Input: part model. Units: mm. Frame: model coordinates. Face numbers are marked on the shaded views. Round coordinates to 2 decimals unless told otherwise and drop trailing zeros. Write each loop counter-clockwise with the first axis right and the second up, starting at its lowest first coordinate (ties: lowest second). Pieces come first, ordered by that corner, then holes. Notation, with made-up numbers: (21.5, 81) -> (30.5, 81) arc R25 cw to (30.5, 97) -> close; hole circle Ø11 at (69, 5.5). An arc over 180 degrees is marked (long way). Use CSV: the item, a comma, the result in double quotes.
```python
from build123d import *

# Parameters (mm, degrees)
BOSS_EXTRUDE1_DEPTH     = 2.8
SKETCH3_W               = 25
SKETCH3_H               = 40
CUT_EXTRUDE1_DEPTH      = 1
SKETCH4_W               = 2.8
SKETCH4_H               = 15
BOSS_EXTRUDE2_DEPTH     = 15
CUT_EXTRUDE2_DEPTH      = 76.211967133
CUT_EXTRUDE2_DEPTH_BACK = 76.211967133
SKETCH5_R               = 2.5


with BuildPart() as part:
    # Sketch2 → Boss-Extrude1 (new body)
    with BuildSketch(Plane(origin=(0, 0, 0), x_dir=(1, 0, 0), z_dir=(0, 1, 0))):
        Polygon((-15, 27.5), (15, 27.5), (15, 7.5), (5, 7.5), (5, 0), (25, 0), (25, -60), (-25, -60), (-25, 0), (-5, 0), (-5, 7.5), (-15, 7.5), align=None)
    extrude(amount=BOSS_EXTRUDE1_DEPTH)

    # Sketch3 → Cut-Extrude1 (cut)
    with BuildSketch(Plane(origin=(0, 2.8, 0), x_dir=(1, 0, 0), z_dir=(0, 1, 0))):
        with Locations((0, -32.5)):
            Rectangle(SKETCH3_W, SKETCH3_H)
    extrude(amount=-CUT_EXTRUDE1_DEPTH, mode=Mode.SUBTRACT)

    # Sketch4 → Boss-Extrude2 (add)
    with BuildSketch(Plane.XZ):
        with Locations((16.4, 30)):
            Rectangle(SKETCH4_W, SKETCH4_H)
        with Locations((-16.4, 30)):
            Rectangle(SKETCH4_W, SKETCH4_H)
    extrude(amount=BOSS_EXTRUDE2_DEPTH)

    # Sketch5 → Cut-Extrude2 (cut, two sides: drawn at the far end of the back side and taken through both)
    with BuildSketch(Plane(origin=(17.8, 0, 0), x_dir=(0, 0, -1), z_dir=(1, 0, 0)).offset(-CUT_EXTRUDE2_DEPTH_BACK)):
        with Locations((-30, -7.5)):
            Circle(SKETCH5_R)
        with BuildLine():
            Line((-22.5, -16.5), (-37.5, -16.5))
            Line((-37.5, -16.5), (-37.5, -7.5))
            ThreePointArc((-37.5, -7.5), (-30, -15), (-22.5, -7.5))
            Line((-22.5, -7.5), (-22.5, -16.5))
        make_face()
    extrude(amount=CUT_EXTRUDE2_DEPTH + CUT_EXTRUDE2_DEPTH_BACK, mode=Mode.SUBTRACT)


solid = part.part
```
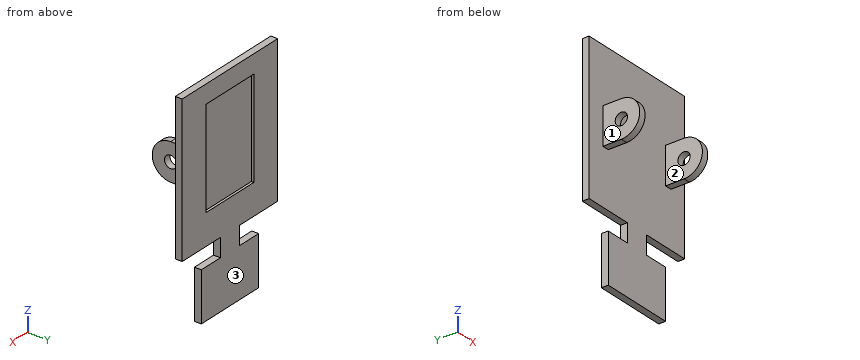
Item 1: Pull-direction query (X, two-part tool) for the marked faces 1, 2 and 3; classes: +X half, -X half, draft (parallel to the pull), parting line (faces both ways), or undercut.
Worked answers:
face 1,"-X half"
face 2,"undercut"
face 3,"draft"
Item 2: Section query B-B on z = 30. Return the cut outline in (x, y), plus the area to 3 significant figures.
Worked answers:
outline,"(-25, 0) -> (-17.8, 0) -> (-17.8, -5) -> (-15, -5) -> (-15, 0) -> (15, 0) -> (15, -5) -> (17.8, -5) -> (17.8, 0) -> (25, 0) -> (25, 2.8) -> (12.5, 2.8) -> (12.5, 1.8) -> (-12.5, 1.8) -> (-12.5, 2.8) -> (-25, 2.8) -> close; (-17.8, -15) -> (-15, -15) -> (-15, -10) -> (-17.8, -10) -> close; (15, -15) -> (17.8, -15) -> (17.8, -10) -> (15, -10) -> close"
area,"171 mm²"
Item 3: Section query D-D on x = 16. Return the cut outline in (y, z), plus the area to 3 significant figures.
Worked answers:
outline,"(-7.5, 22.5) -> (0, 22.5) -> (0, 0) -> (2.8, 0) -> (2.8, 60) -> (0, 60) -> (0, 37.5) -> (-7.5, 37.5) arc R7.5 ccw to start; hole circle Ø5 at (-7.5, 30)"
area,"349 mm²"
Item 4: Line query: line 1 (Z direction, x = 16.3, y = -7.5); line 2 (Y direction, x = 17.25, z = 30); line 3 (X direction, y = -7.25, z = 36). Output: solid intervals per line, ascending.
Worked answers:
line 1,"z = 22.5 to 27.5, 32.5 to 37.5"
line 2,"y = -15 to -10, -5 to 2.8"
line 3,"x = -17.8 to -15, 15 to 17.8"
Item 5: First-contact query: pin 1 Ø3 at (x, y) = (17.5, 1.5) entering from -Z; pin 2 Ø0.8 at (x, y) = (-16, -3.5) entering from -Z; pin 3 Ø2 at (y, z) = (1, -3.5) entering from -X. Flat tips, straight axial feed; report the tip coordinate or a pass-through.
Worked answers:
pin 1,"stops at z = 0"
pin 2,"stops at z = 22.5"
pin 3,"stops at x = -5"
Item 6: Section query A-A on x = -11. Return the cut outline in (y, z).
Worked answers:
outline,"(0, -27.5) -> (2.8, -27.5) -> (2.8, -7.5) -> (0, -7.5) -> close; (0, 0) -> (2.8, 0) -> (2.8, 12.5) -> (1.8, 12.5) -> (1.8, 52.5) -> (2.8, 52.5) -> (2.8, 60) -> (0, 60) -> close"
Item 7: Section query C-C on y = -2.5. Return the cut outline in (x, z), plus the area to 3 significant figures.
Worked answers:
outline,"(-17.8, 22.5) -> (-15, 22.5) -> (-15, 37.5) -> (-17.8, 37.5) -> close; (15, 22.5) -> (17.8, 22.5) -> (17.8, 37.5) -> (15, 37.5) -> close"
area,"84.0 mm²"
